from build123d import *

# Parameters (mm, degrees)
SKETCH_1_W          = 50
SKETCH_1_H          = 40
EXTRUDE_1_DEPTH     = 4
SKETCH_2_R          = 1.75
CUT_EXTRUDE_1_DEPTH = 4
SKETCH_3_W          = 4
SKETCH_3_H          = 40
CUT_EXTRUDE_2_DEPTH = 12
SKETCH_8_W          = 16
SKETCH_8_H          = 10
SKETCH_11_W         = 16
SKETCH_11_H         = 10


with BuildPart() as part:
    # 草图1 → 凸台-拉伸1 (new body)
    with BuildSketch(Plane.XY):
        Rectangle(SKETCH_1_W, SKETCH_1_H)
    extrude(amount=EXTRUDE_1_DEPTH)

    # 草图2 → 切除-拉伸1 (cut)
    with BuildSketch(Plane.XY.offset(4)):
        with Locations((-20.5, 15)):
            Circle(SKETCH_2_R)
        with Locations((-4.5, 15)):
            Circle(SKETCH_2_R)
        with Locations((20.5, 15)):
            Circle(SKETCH_2_R)
        with Locations((20.5, -15)):
            Circle(SKETCH_2_R)
        with Locations((4.5, -15)):
            Circle(SKETCH_2_R)
        with Locations((-20.5, -15)):
            Circle(SKETCH_2_R)
    extrude(amount=-CUT_EXTRUDE_1_DEPTH, mode=Mode.SUBTRACT)

    # 草图3 → 切除-拉伸2 (cut)
    with BuildSketch(Plane.ZY.offset(25)):
        with Locations((2, 0)):
            Rectangle(SKETCH_3_W, SKETCH_3_H)
    extrude(amount=-CUT_EXTRUDE_2_DEPTH, mode=Mode.SUBTRACT)

    # 草图8 → 切除-放样5 section 0
    with BuildSketch(Plane.XY):
        with Locations((18, 0)):
            Rectangle(SKETCH_8_W, SKETCH_8_H)
    # 草图11 → 切除-放样5 section 1
    with BuildSketch(Plane.XY.offset(4)):
        with Locations((17.972560725, 0.020424216)):
            Rectangle(SKETCH_11_W, SKETCH_11_H)
    loft(mode=Mode.SUBTRACT)


solid = part.part
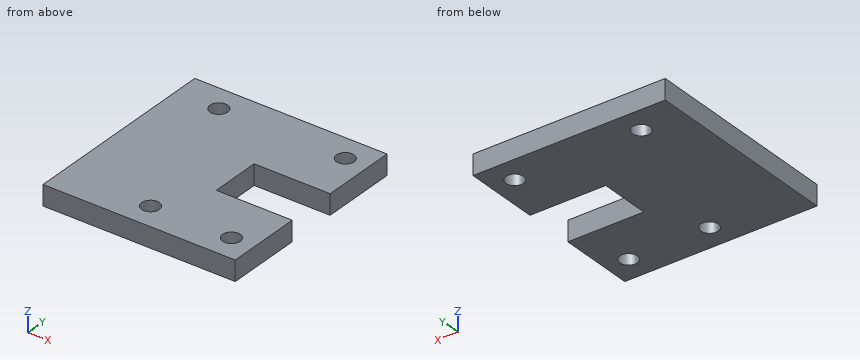
The model under review builds one solid part; all positions refer to its coordinate system, in mm. Give positions to 0.01 mm unless a question says otherwise; leave off trailing zeros. Loops run counter-clockwise (first coordinate to the right, second up) from the corner with the lowest first, then second, coordinate; pieces in that order, holes last. Notation, with made-up numbers: (-31, 59.25) -> (-1, 59.25) arc R15 cw to (-1, 85.25) -> close; hole circle Ø8 at (-34, -11.5). An arc over 180 degrees is marked (long way). Answer as a JSON object with one key per item and string values. Group by question number.
Q1. Take a section at B-B (y = -15). Write out the cut boundary in (x, z).
Q2. Wall thickness on line 1 along Y through (x, z) = (20.5, 0.85); line 2 along Y through (x, z) = (10.5, 2.45); line 3 along Y through (x, z) = (-4.5, 3.25): over which ranges is each line inside the solid? List them lowest first.
Q3. Take a section at A-A (x = 4.5). Write out the cut boundary in (y, z), plus the area to 3 significant figures.
Q4. Take a section at C-C (x = 20.5). State how many separate pieces and enclosed holes the cut face has, plus the area to 3 significant figures.
Answer below:
{
 "1": {"outline": "(-13, 0) -> (2.75, 0) -> (2.75, 4) -> (-13, 4) -> close; (6.25, 0) -> (18.75, 0) -> (18.75, 4) -> (6.25, 4) -> close; (22.25, 0) -> (25, 0) -> (25, 4) -> (22.25, 4) -> close"},
 "2": {"line 1": "y = -20 to -16.75, -13.25 to -5, 5 to 13.25, 16.75 to 20", "line 2": "y = -20 to -4.99, 5.01 to 20", "line 3": "y = -20 to 13.25, 16.75 to 20"},
 "3": {"outline": "(-20, 0) -> (-16.75, 0) -> (-16.75, 4) -> (-20, 4) -> close; (-13.25, 0) -> (20, 0) -> (20, 4) -> (-13.25, 4) -> close", "area": "146 mm2"},
 "4": {"separate pieces": "4", "enclosed holes": "0", "area": "92.0 mm2"}
}
